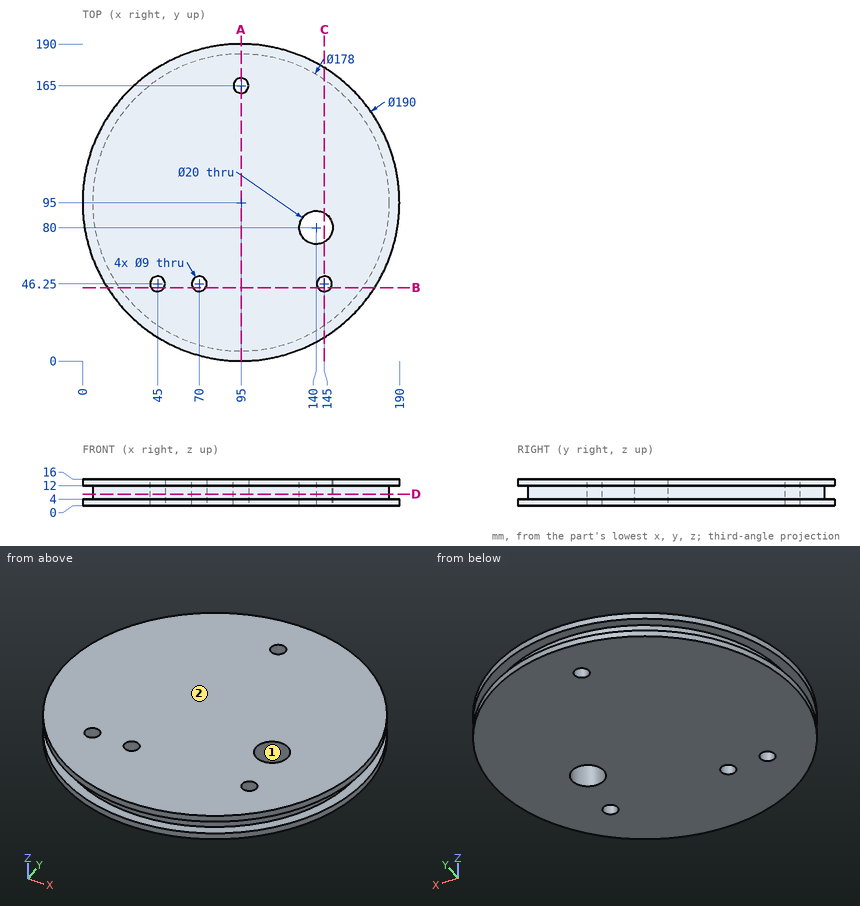
Answer from the drawing. Dimensions are ordinates in mm from the lowest x, y and z of the part. Coordinates: 2 decimals unless noted, no trailing zeros. Write each loop counter-clockwise with the first axis right and the second up, starting at its lowest first coordinate (ties: lowest second). Pieces come first, ordered by that corner, then holes. Notation, with made-up numbers: (-8, -26) - (24, -26) arc R8 cw to (24, -19) - close; hole circle Ø10 at (-17, 66). An arc over 180 degrees is marked (long way). Return JSON: item names as keys, results as strings. Group by question number.
Q1. For a pull along X with two mould halves and no side action, classify the marked faces 1 and 2 as +X half, -X half, draft (parallel to the pull), parting line (faces both ways), or undercut.
Q2. The part is cut by section D-D on z = 7. Write down the section's boundary in (x, y), and give its area (3 significant figures).
Q3. The part is cut by section A-A on x = 95. Write down the section's boundary in (y, z).
Q4. The part is cut by section B-B on y = 44. Write down the section's boundary in (x, z), and give its area (3 significant figures).
Q5. Find the intervals of material crossed by line 1 along Z through (x, y) = (59.5, 10); line 2 along X through (y, z) = (46.5, 3.25); line 3 along X through (y, z) = (88.5, 8.75), in increasing order. Write a range as [from, to].
Q6. Flat-ended cylindrical pins translate along their axes: pin 1 Ø3 at (x, z) = (108, 4) entering from -Y; pin 2 Ø7 at (x, y) = (70, 46.25) entering from +Z; pin 3 Ø1.5 at (y, z) = (111.5, 4) entering from +X; pin 4 Ø1.5 at (y, z) = (46.5, 5.5) entering from +X. Find the tip coordinate at first contact, or state that the pin passes through.
Q7. The part is cut by section C-C on x = 145. Write down the section's boundary in (y, z), and give its area (3 significant figures).
Evaluation:
{
 "1": {"face 1": "undercut", "face 2": "draft"},
 "2": {"outline": "circle Ø178 at (95, 95); hole circle Ø9 at (45, 46.25); hole circle Ø9 at (70, 46.25); hole circle Ø9 at (95, 165); hole circle Ø20 at (140, 80); hole circle Ø9 at (145, 46.25)", "area": "24,300 mm2"},
 "3": {"outline": "(0, 0) - (160.5, 0) - (160.5, 16) - (0, 16) - (0, 12) - (6, 12) - (6, 4) - (0, 4) - close; (169.5, 0) - (190, 0) - (190, 4) - (184, 4) - (184, 12) - (190, 12) - (190, 16) - (169.5, 16) - close"},
 "4": {"outline": "(14.85, 0) - (41.1, 0) - (41.1, 16) - (14.85, 16) - (14.85, 12) - (22.06, 12) - (22.06, 4) - (14.85, 4) - close; (48.9, 0) - (66.1, 0) - (66.1, 16) - (48.9, 16) - close; (73.9, 0) - (141.1, 0) - (141.1, 16) - (73.9, 16) - close; (148.9, 0) - (175.15, 0) - (175.15, 4) - (167.94, 4) - (167.94, 12) - (175.15, 12) - (175.15, 16) - (148.9, 16) - close", "area": "2,080 mm2"},
 "5": {"line 1": "z = [0, 4], [12, 16]", "line 2": "x = [13.31, 40.51], [49.49, 65.51], [74.49, 140.51], [149.49, 176.69]", "line 3": "x = [6.24, 134.73], [145.27, 183.76]"},
 "6": {"pin 1": "stops at y = 0.7", "pin 2": "passes through", "pin 3": "stops at x = 188.69", "pin 4": "stops at x = 170.11"},
 "7": {"outline": "(14.22, 0) - (41.75, 0) - (41.75, 16) - (14.22, 16) - (14.22, 12) - (21.37, 12) - (21.37, 4) - (14.22, 4) - close; (50.75, 0) - (71.34, 0) - (71.34, 16) - (50.75, 16) - close; (88.66, 0) - (175.78, 0) - (175.78, 4) - (168.63, 4) - (168.63, 12) - (175.78, 12) - (175.78, 16) - (88.66, 16) - close", "area": "2,050 mm2"}
}
